```python
from build123d import *

# Parameters (mm, degrees)
BOSS_EXTRUDE1_DEPTH = 101.6


with BuildPart() as part:
    # Sketch1 → Boss-Extrude1 (new body)
    with BuildSketch(Plane.XY):
        with BuildLine():
            Line((-38.109310446, 0), (-38.109310446, 12.319))
            Line((-38.109310446, 12.319), (38.11716556, 12.319))
            Line((38.11716556, 12.319), (38.11716556, 0))
            Line((38.11716556, 0), (17.238227932, 0))
            ThreePointArc((17.238227932, 0), (15.959298514, -6.515926117), (12.312281561, -12.065))
            Line((12.312281561, -12.065), (12.05814004, -12.065))
            Line((12.05814004, -12.065), (-12.05814004, -12.065))
            Line((-12.05814004, -12.065), (-12.312281561, -12.065))
            ThreePointArc((-12.312281561, -12.065), (-15.959298514, -6.515926117), (-17.238227932, 0))
            Line((-17.238227932, 0), (-38.109310446, 0))
        make_face()
        with BuildLine():
            Line((-7.459501807, 7.931540852), (7.459501807, 7.931540852))
            ThreePointArc((7.459501807, 7.931540852), (10.887932539, 0.08020301), (7.575537086, -7.820789305))
            Line((7.575537086, -7.820789305), (-7.575537086, -7.820789305))
            ThreePointArc((-7.575537086, -7.820789305), (-10.887932539, 0.08020301), (-7.459501807, 7.931540852))
        make_face(mode=Mode.SUBTRACT)
    extrude(amount=-BOSS_EXTRUDE1_DEPTH)


solid = part.part
```
Design review of the part built by this model. Coordinates are the model's own, in mm. A direction names the side the tool comes from. Coordinates: 2 decimals unless noted, no trailing zeros. Loops run counter-clockwise (first coordinate to the right, second up) from the corner with the lowest first, then second, coordinate; pieces in that order, holes last.
Q1. We need section A-A on x = -4. State the section outline as (y, z) points (3 decimals).
Reported:
outline: (-12.065, -101.6) - (-7.821, -101.6) - (-7.821, 0) - (-12.065, 0) - close; (7.932, -101.6) - (12.319, -101.6) - (12.319, 0) - (7.932, 0) - close
Q2. To check wall thickness, follow line 1 (Y direction, x = 6.5, z = -74.5) (3 decimals); line 2 (X direction, y = 0.25, z = -69); line 3 (X direction, y = -0.25, z = -29.5). State the ranges of each line that lie inside material, in increasing order.
Reported:
line 1: y = -12.065 to -7.821, 7.932 to 12.319
line 2: x = -38.11 to -10.89, 10.89 to 38.12
line 3: x = -17.24 to -10.89, 10.89 to 17.24
Q3. Tool access review of faces 1 (the face through (0, 7.932, -50)), 2 (the face through (0.5, 8.4, 0)), 3 (the face through (-28, 0, -50)): name each direction out of +Z, -Z, +X, -X, +Y, -Y from which nothing blocks a thin tool from reaching the whole face with its end or side.
Reported:
face 1: +Z, -Z
face 2: +Z, +X, -X, +Y, -Y
face 3: +Z, -Z, -X, -Y
Q4. We need section D-D on x = -21.5. State the section outline as (y, z) points.
Reported:
outline: (0, -101.6) - (12.32, -101.6) - (12.32, 0) - (0, 0) - close
Q5. We need section C-C on z = -71. State the section outline as (x, y) points (1 decimal).
Reported:
outline: (-38.1, 0) - (-17.2, 0) arc R17.2 ccw to (-12.3, -12.1) - (12.3, -12.1) arc R17.2 ccw to (17.2, 0) - (38.1, 0) - (38.1, 12.3) - (-38.1, 12.3) - close; hole (-7.6, -7.8) - (7.6, -7.8) arc R10.9 ccw to (7.5, 7.9) - (-7.5, 7.9) arc R10.9 ccw to start
Q6. The part is to be moulded in two halves that separate along Y. For faces 4 (the face through (38.117, 6, -50)), 5 (the face through (0, -7.821, -50)), 6 (the face through (28, 0, -50)), say which applies: +Y half, -Y half, draft (parallel to the pull), parting line (faces both ways), or undercut.
Reported:
face 4: draft
face 5: undercut
face 6: -Y half
Q7. For pin 1 (8 mm diameter, centred on x = -21, y = -2.5, fed in from +Z); pin 2 (10.5 mm diameter, centred on x = -30, z = -72, fed in from -Y); pin 3 (4 mm diameter, centred on y = -2.5, z = -16, fed in from -X), all flat-tipped, find the tip position at first contact; note any pin that passes through.
Reported:
pin 1: stops at z = 0
pin 2: stops at y = 0
pin 3: stops at x = -17.23
Q8. We need section B-B on y = -5. State the section outline as (x, z) points, and give its area (3 significant figures).
Reported:
outline: (-16.5, -101.6) - (-9.67, -101.6) - (-9.67, 0) - (-16.5, 0) - close; (9.67, -101.6) - (16.5, -101.6) - (16.5, 0) - (9.67, 0) - close
area: 1,390 mm2
